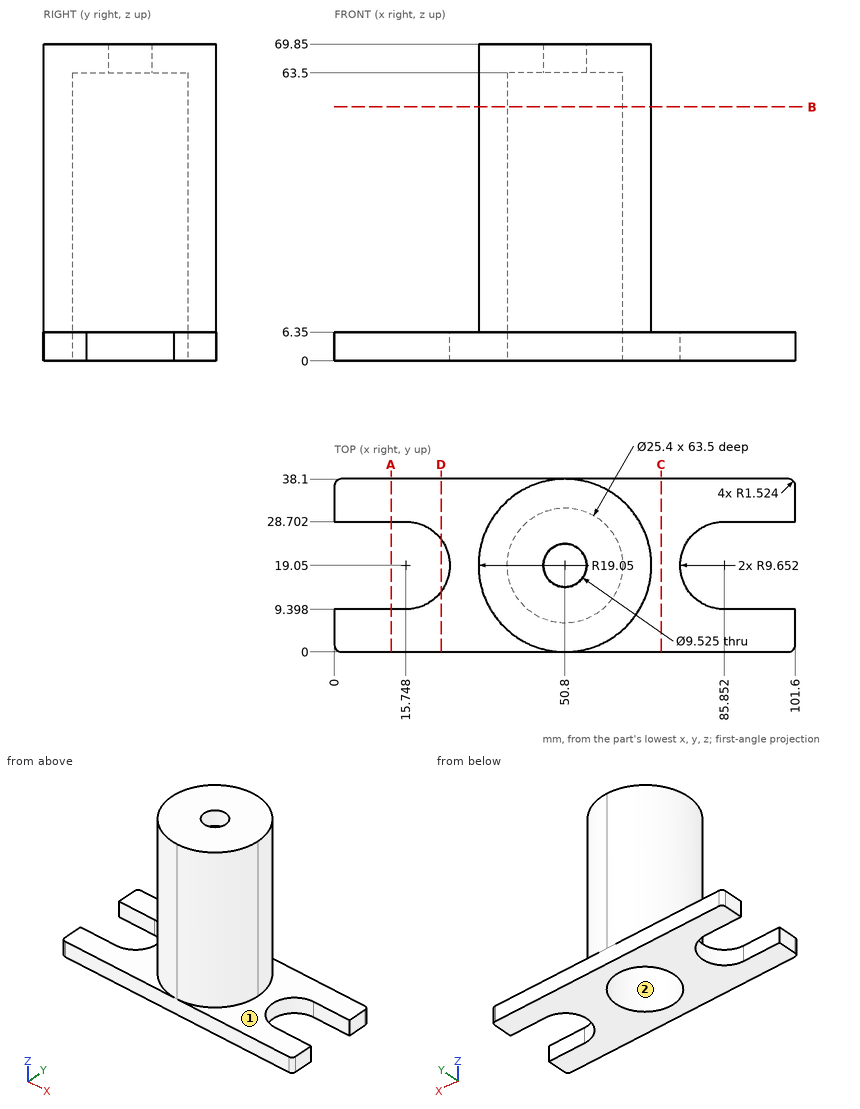
The figure shows three views and two pictorial views of one solid part (mm, origin at its lowest corner). Answer the questions. Coordinates: 2 decimals unless noted, no trailing zeros. Loops run counter-clockwise (first coordinate to the right, second up) from the corner with the lowest first, then second, coordinate; pieces in that order, holes last.
1) Find the intervals of material crossed by L1, parallel to Y at x = 89, z = 5; L2, parallel to Y at x = 50, z = 42; L3, parallel to X at y = 19, z = 37, in increasing order.
2) Find section C-C on x = 72. Write down the section's boundary in (y, z), then the cut area to 3 significant figures.
3) Find section D-D on x = 23.5. Write down the section's boundary in (y, z).
4) Find section B-B on z = 56. Write down the section's boundary in (x, y), then the cut area to 3 significant figures.
5) Determine the mould class of the marked faces 1 and 2 for opening direction Y: pulls with the +Y half, pulls with the -Y half, needs draft (parallel to the pull), parting line crosses it, or undercut.
6) Flat-ended cylindrical pins translate along their axes: pin 1 Ø12.5 at (x, y) = (54.5, 22) entering from -Z; pin 2 Ø10 at (y, z) = (26.5, 15.5) entering from +X; pin 3 Ø2 at (y, z) = (19, 17) entering from +X; pin 4 Ø7.5 at (x, y) = (50.8, 19.05) entering from -Z. Find the tip coordinate at first contact, or state that the pin passes through.
7) Find section A-A on x = 12.5. Write down the section's boundary in (y, z).
Values:
1. L1: y = 0 to 9.4, 28.7 to 38.1
1. L2: y = 0.02 to 6.38, 31.72 to 38.08
1. L3: x = 31.75 to 38.1, 63.5 to 69.85
2. outline: (0, 0) - (38.1, 0) - (38.1, 6.35) - (0, 6.35) - close
2. area: 242 mm2
3. outline: (0, 0) - (13.3, 0) - (13.3, 6.35) - (0, 6.35) - close; (24.8, 0) - (38.1, 0) - (38.1, 6.35) - (24.8, 6.35) - close
4. outline: (50.8, 0) arc R19.05 ccw to (69.85, 19.05) arc R19.05 ccw (long way) to start; hole circle Ø25.4 at (50.8, 19.05)
4. area: 633 mm2
5. face 1: needs draft
5. face 2: undercut
6. pin 1: stops at z = 63.5
6. pin 2: stops at x = 69.69
6. pin 3: stops at x = 69.85
6. pin 4: passes through
7. outline: (0, 0) - (9.4, 0) - (9.4, 6.35) - (0, 6.35) - close; (28.7, 0) - (38.1, 0) - (38.1, 6.35) - (28.7, 6.35) - close
